Input: part model. Units: mm. Frame: model coordinates. A direction names the side the tool comes from. Give positions to 0.01 mm unless a question says otherwise; leave off trailing zeros. Order: outer loops, then holes, each group sorted by start corner. A loop starts at its lowest first (then second) coordinate and runs counter-clockwise, first axis right, second up.
```python
from build123d import *

# Parameters (mm, degrees)
F0_W     = 400
F0_H     = 400
F1_DEPTH = 3
F2_R     = 1.25
F2_W     = 12
F2_H     = 2
F3_DEPTH = 2
F4_DEPTH = 2


with BuildPart() as f1:
    # F0 (on Top) → F1 (new body)
    with BuildSketch(Plane.XY):
        Rectangle(F0_W, F0_H)
    extrude(amount=-F1_DEPTH)

    # F2 (on Right) → F3 (join)
    with BuildSketch(Plane.YZ):
        with BuildLine():
            ThreePointArc((-3.4732674635, 10.0854136027), (-6, 11.75), (-8.5267325365, 10.0854136027))
            ThreePointArc((-8.5267325365, 10.0854136027), (-6.5540692757, 6.3063951222), (-3.25, 9))
            ThreePointArc((-3.25, 9), (-3.3063951222, 9.5540692757), (-3.4732674635, 10.0854136027))
        make_face()
        with Locations((-6, 9)):
            Circle(F2_R, mode=Mode.SUBTRACT)
        with BuildLine():
            Line((-8.5267325365, 10.0854136027), (-12, 2))
            Line((-12, 2), (0, 2))
            Line((0, 2), (-3.4732674635, 10.0854136027))
            ThreePointArc((-3.4732674635, 10.0854136027), (-3.3063951222, 9.5540692757), (-3.25, 9))
            ThreePointArc((-3.25, 9), (-6.5540692757, 6.3063951222), (-8.5267325365, 10.0854136027))
        make_face()
        with Locations((-6, 1)):
            Rectangle(F2_W, F2_H)
        with Locations((6, 1)):
            Rectangle(F2_W, F2_H)
        with BuildLine():
            Line((3.4732674635, 10.0854136027), (0, 2))
            Line((0, 2), (12, 2))
            Line((12, 2), (8.5267325365, 10.0854136027))
            ThreePointArc((8.5267325365, 10.0854136027), (8.6936048778, 9.5540692757), (8.75, 9))
            ThreePointArc((8.75, 9), (5.4459307243, 6.3063951222), (3.4732674635, 10.0854136027))
        make_face()
        with BuildLine():
            ThreePointArc((8.5267325365, 10.0854136027), (6, 11.75), (3.4732674635, 10.0854136027))
            ThreePointArc((3.4732674635, 10.0854136027), (5.4459307243, 6.3063951222), (8.75, 9))
            ThreePointArc((8.75, 9), (8.6936048778, 9.5540692757), (8.5267325365, 10.0854136027))
        make_face()
        with Locations((6, 9)):
            Circle(F2_R, mode=Mode.SUBTRACT)
    extrude(amount=F3_DEPTH)

    # F4 (add): a face of the model
    f4_faces = [f1.faces().sort_by_distance(p)[0] for p in [
        (0, -6, 11.4827805209),
    ]]
    extrude(f4_faces, amount=F4_DEPTH)


solid = f1.part
```
1) Reachability of faces 1 (the face through (-3, 3, -3)), 2 (the face through (-2, -0.2, 2)), 3 (the face through (2, -0.2, 2)) from +Z, -Z, +X, -X, +Y, -Y: full face, straight path, thin tool, end or side. Return the list, or none.
2) Cut plane A-A (z = 5.25). Return the cut outline in (x, y).
3) First-contact query: P1, Ø1.6, axis at x = 0, z = 1, coming from the +Y side; P2, Ø10, axis at x = 111.5, y = -76.5, coming from the +Z side; P3, Ø0.6, axis at x = 0.5, z = 1, coming from the -Y side; P4, Ø2, axis at x = -90, z = 2.5, coming from the -Y side. Flat tips, straight axial feed; report the tip coordinate or a pass-through.
4) Line query: probe 1 along Z at (x, y) = (0.65, -6); probe 2 along Z at (x, y) = (-111, 112). Output: solid intervals per line, ascending.
5) Cut plane B-B (x = 140). Return the cut outline in (y, z), then the cut area to 3 significant figures.
Geometry says:
1. face 1: -Z, +X, -X, +Y, -Y
1. face 2: +Z, -X, +Y, -Y
1. face 3: +Z, +X, +Y, -Y
2. outline: (-2, -10.6) - (2, -10.6) - (2, -1.4) - (-2, -1.4) - close; (-2, 1.4) - (2, 1.4) - (2, 10.6) - (-2, 10.6) - close
3. P1: stops at y = 12
3. P2: stops at z = 0
3. P3: stops at y = -12
3. P4: passes through
4. probe 1: z = -3 to 7.75, 10.25 to 11.75
4. probe 2: z = -3 to 0
5. outline: (-200, -3) - (200, -3) - (200, 0) - (-200, 0) - close
5. area: 1,200 mm2
